from build123d import *

# Parameters (mm, degrees)
BOSS_EXTRUDE1_DEPTH      = 99.06
BOSS_EXTRUDE1_DEPTH_BACK = 1.016
SKETCH2_R                = 3
SKETCH2_R_2              = 10
SKETCH2_R_3              = 5
SKETCH2_W                = 36
SKETCH2_H                = 47
CUT_EXTRUDE1_DEPTH       = 194.478154064


with BuildPart() as part:
    # Sketch1 → Boss-Extrude1 (new, two sides: drawn at the far end of the back side and taken through both)
    with BuildSketch(Plane.XY.offset(-BOSS_EXTRUDE1_DEPTH_BACK)):
        Polygon((165.1, -13.97), (78.74, -13.97), (66.04, 2.54), (0, 2.54), (0, 0), (66.04, 0), (78.74, -16.51), (165.1, -16.51), align=None)
    extrude(amount=BOSS_EXTRUDE1_DEPTH + BOSS_EXTRUDE1_DEPTH_BACK)

    # Sketch2 → Cut-Extrude1 (cut, through all)
    with BuildSketch(Plane(origin=(0, 2.54, 0), x_dir=(1, 0, 0), z_dir=(0, 1, 0))):
        with Locations(Location((85, -7.584, 0), (0, 0, 270))):
            Circle(SKETCH2_R)
        with Locations(Location((85, -83.384, 0), (0, 0, 270))):
            Circle(SKETCH2_R)
        with Locations(Location((149.6, -30.584, 0), (0, 0, 270))):
            Circle(SKETCH2_R)
        with Locations(Location((14.5, -45.484, 0), (0, 0, 270))):
            Circle(SKETCH2_R_2)
        with Locations(Location((142, -44.584, 0), (0, 0, 270))):
            Circle(SKETCH2_R_3)
        with Locations((46, -45.484)):
            Rectangle(SKETCH2_W, SKETCH2_H)
    extrude(amount=-CUT_EXTRUDE1_DEPTH, mode=Mode.SUBTRACT)


solid = part.part
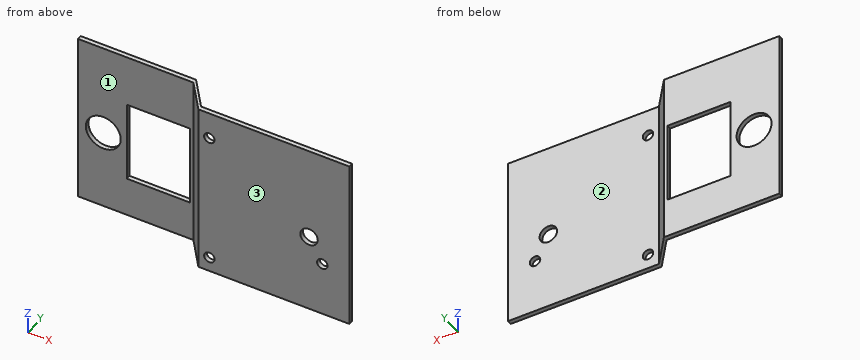
For this review, take the finished solid that the model builds, in its own axes (mm). Face numbers are marked on the shaded views. A direction names the side the tool comes from. Round coordinates to 2 decimals unless told otherwise and drop trailing zeros. Loops run counter-clockwise (first coordinate to the right, second up) from the corner with the lowest first, then second, coordinate; pieces in that order, holes last. Notation, with made-up numbers: (-14, 27) - (14, 27) arc R29 ccw to (14, 58) - close; hole circle Ø7 at (87, -40). An arc over 180 degrees is marked (long way). Answer as CSV lines item,"result".
(1) Tool access review of the marked faces 1, 2 and 3: name each direction out of +Z, -Z, +X, -X, +Y, -Y from which nothing blocks a thin tool from reaching the whole face with its end or side.
Checked values:
face 1,"+Z, -Z, -X, -Y"
face 2,"+Z, -Z, +X, +Y"
face 3,"+Z, -Z, +X, -X, -Y"
(2) Wall thickness on line 1 (Z direction, x = 149.6, y = -15.1); line 2 (Y direction, x = 46, z = 8.5); line 3 (Y direction, x = 124, z = 82): over which ranges is each line inside the solid? List them lowest first.
Checked values:
line 1,"z = -1.02 to 27.58, 33.58 to 99.06"
line 2,"y = 0 to 2.54"
line 3,"y = -16.51 to -13.97"
(3) Insertion check: P1, Ø1, axis at x = 85.5, z = 78, coming from the +Y side; P2, Ø0.8, axis at y = 1, z = 50, coming from the +X side; P3, Ø3, axis at y = -10, z = 86.5, coming from the +X side. Each pin has a flat end and moves straight along its axis. Give the tip position at first contact, or say it passes through.
Checked values:
P1,"stops at y = -13.97"
P2,"stops at x = 67.53"
P3,"stops at x = 76.84"
(4) Consider section D-D on x = 149.6. Give the boundary of the cut face in (y, z), then the cut area to 3 significant figures.
Checked values:
outline,"(-16.51, -1.02) - (-13.97, -1.02) - (-13.97, 27.58) - (-16.51, 27.58) - close; (-16.51, 33.58) - (-13.97, 33.58) - (-13.97, 99.06) - (-16.51, 99.06) - close"
area,"239 mm2"
(5) Consider section A-A on x = 60. Give the boundary of the cut face in (y, z).
Checked values:
outline,"(0, -1.02) - (2.54, -1.02) - (2.54, 21.98) - (0, 21.98) - close; (0, 68.98) - (2.54, 68.98) - (2.54, 99.06) - (0, 99.06) - close"
(6) Consider section B-B on x = 85. Give the boundary of the cut face in (y, z), then the cut area to 3 significant figures.
Checked values:
outline,"(-16.51, -1.02) - (-13.97, -1.02) - (-13.97, 4.58) - (-16.51, 4.58) - close; (-16.51, 10.58) - (-13.97, 10.58) - (-13.97, 80.38) - (-16.51, 80.38) - close; (-16.51, 86.38) - (-13.97, 86.38) - (-13.97, 99.06) - (-16.51, 99.06) - close"
area,"224 mm2"
(7) Consider section C-C on z = 16.5. Give the boundary of the cut face in (x, y), then the cut area to 3 significant figures.
Checked values:
outline,"(0, 0) - (66.04, 0) - (78.74, -16.51) - (165.1, -16.51) - (165.1, -13.97) - (78.74, -13.97) - (66.04, 2.54) - (0, 2.54) - close"
area,"419 mm2"
